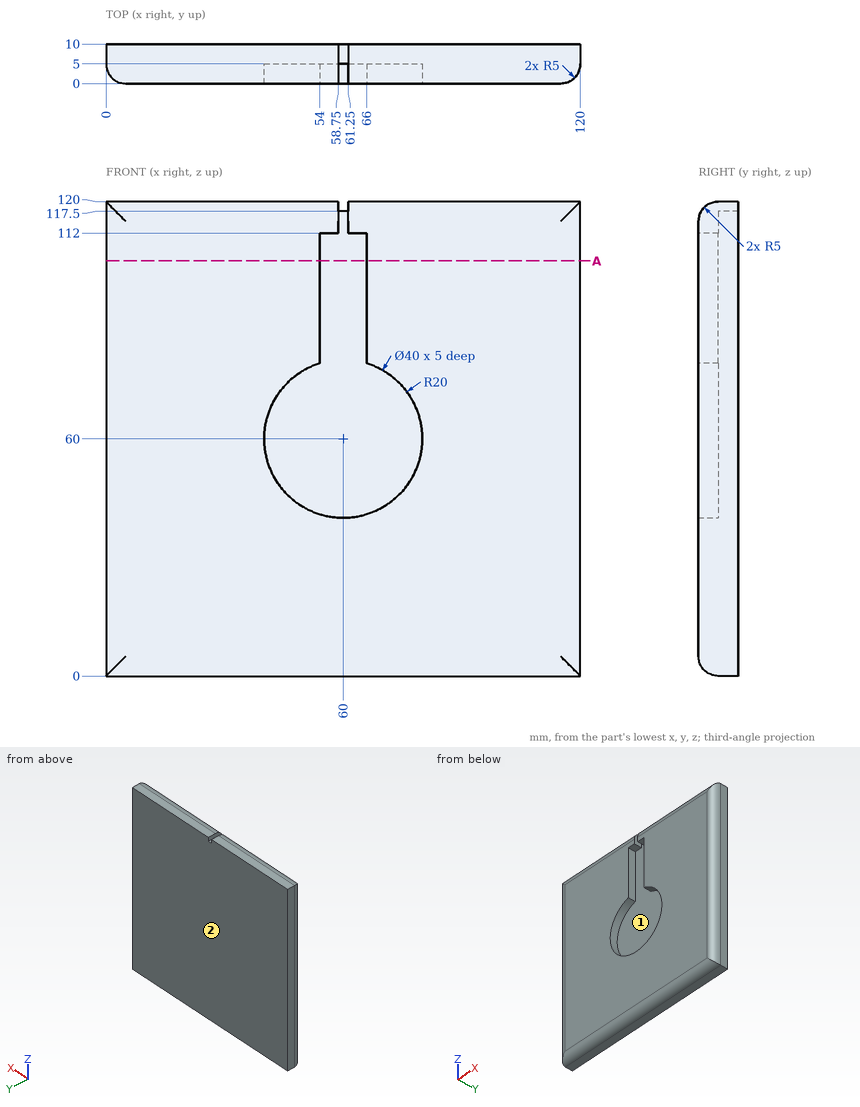
Print and shaded views of the part. All mm, measured from the part's lowest x, y and z. Coordinates: 2 decimals unless noted, no trailing zeros. Write each loop counter-clockwise with the first axis right and the second up, starting at its lowest first coordinate (ties: lowest second). Pieces come first, ordered by that corner, then holes.
(1) Two-plate mould, pull along Z, no slides. Class the marked faces 1 and 2: +Z half, -Z half, draft (parallel to the pull), parting line (faces both ways), or undercut.
(2) Flat gauge pins, fed straight in: pin 1 (12 mm diameter, centred on x = 60.5, z = 19, fed in from -Y); pin 2 (2 mm diameter, centred on y = 1.5, z = 24.5, fed in from +X); pin 3 (1.4 mm diameter, centred on x = 63, y = 2, fed in from -Z); pin 4 (2 mm diameter, centred on x = 60, y = 8.5, fed in from +Z). Where does each tip first touch, or does it go through?
(3) Cut at A-A, the plane z = 105. List the corners of the cut face in (x, y), and give its area (3 significant figures).
(4) Drill centre lines: probe 1 along Y at (x, z) = (66.5, 59.5); probe 2 along Z at (x, y) = (47.5, 1.5); probe 3 along X at (y, z) = (1.9, 60). Where is each one in solid material? Low to high.
Geometry says:
1. face 1: undercut
1. face 2: draft
2. pin 1: stops at y = 0
2. pin 2: stops at x = 119.33
2. pin 3: stops at z = 0.56
2. pin 4: stops at z = 117.5
3. outline: (0, 5) arc R5 ccw to (5, 0) - (54, 0) - (54, 5) - (66, 5) - (66, 0) - (115, 0) arc R5 ccw to (120, 5) - (120, 10) - (0, 10) - close
3. area: 1,130 mm2
4. probe 1: y = 5 to 10
4. probe 2: z = 1.43 to 44.39, 75.61 to 118.57
4. probe 3: x = 1.08 to 40, 80 to 118.92
